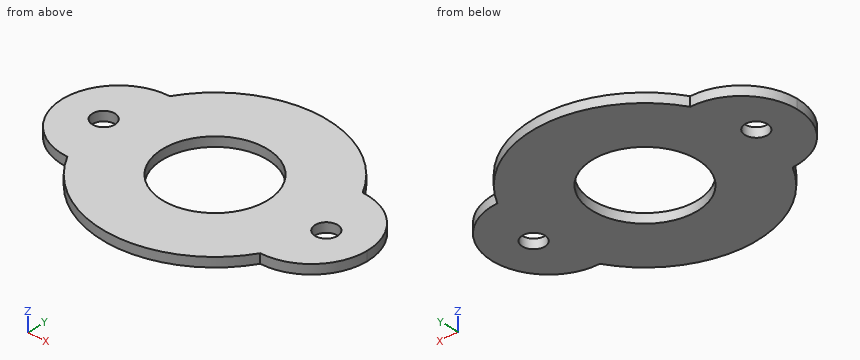
from build123d import *

# Parameters (mm, degrees)
F0_R     = 7
F1_DEPTH = 1.25
F2_R     = 7.49999
F3_D     = 3


# Not quite as in the source:
# - a fillet or chamfer is up to 0.001 mm smaller than in the source, because OpenCascade refuses the exact size


with BuildPart() as f1:
    # F0 (on Top) → F1 (new body)
    with BuildSketch(Plane.XY):
        with BuildLine():
            ThreePointArc((-12.990381, -7.5), (-15, 0), (-12.990381, 7.5))
            Line((-12.990381, 7.5), (-20.490381, 7.5))
            Line((-20.490381, 7.5), (-20.490381, -7.5))
            Line((-20.490381, -7.5), (-12.990381, -7.5))
        make_face()
        with BuildLine():
            ThreePointArc((12.990381, -7.5), (14.488887, -3.882286), (15, 0))
            ThreePointArc((15, 0), (14.488887, 3.882286), (12.990381, 7.5))
            ThreePointArc((12.990381, 7.5), (0, 15), (-12.990381, 7.5))
            ThreePointArc((-12.990381, 7.5), (-15, 0), (-12.990381, -7.5))
            ThreePointArc((-12.990381, -7.5), (0, -15), (12.990381, -7.5))
        make_face()
        Circle(F0_R, mode=Mode.SUBTRACT)
        with BuildLine():
            ThreePointArc((12.990381, 7.5), (14.488887, 3.882286), (15, 0))
            ThreePointArc((15, 0), (14.488887, -3.882286), (12.990381, -7.5))
            Line((12.990381, -7.5), (20.490381, -7.5))
            Line((20.490381, -7.5), (20.490381, 7.5))
            Line((20.490381, 7.5), (12.990381, 7.5))
        make_face()
    extrude(amount=F1_DEPTH)

    # F2 (radius 7.5 in the source; OpenCascade refuses exactly that, so slightly less here)
    f2_edges = [f1.edges().sort_by_distance(p)[0] for p in [
        (-20.490381, 7.5, 0.625),
        (-20.490381, -7.5, 0.625),
        (20.490381, 7.5, 0.625),
        (20.490381, -7.5, 0.625),
    ]]
    fillet(f2_edges, radius=F2_R)

    # F3 (through all)
    with Locations(Plane(origin=(0, 0, 0), x_dir=(1, 0, 0), z_dir=(0, 0, -1))):
        with Locations((15, 0), (-15, 0)):
            Hole(F3_D / 2)


solid = f1.part
CAD build for the part. Positions are in the model's coordinates, mm. Coordinates: 2 decimals unless noted, no trailing zeros. Write each loop counter-clockwise with the first axis right and the second up, starting at its lowest first coordinate (ties: lowest second). Pieces come first, ordered by that corner, then holes. Notation, with made-up numbers: M 6,53.25 L 14,53.25 A24 cw 14,78.25 Z; hole C 10,53.25 d6. An arc over 180 degrees is marked long. Answer as a JSON object with one key per item and string values. Group by question number.
1) Pin check, flat tip, straight feed: pin 1 Ø3 at (x, y) = (-7, 11.5) entering from -Z. Stop position of the tip, or through.
2) Saw through at A-A (x = 0). Write the cut outline in (y, z).
3) Saw through at C-C (y = 12). Write the cut outline in (x, z), plus the area to 3 significant figures.
4) Saw through at B-B (z = 0.5). Give the number of separate pieces and of enclosed holes in the cut face, plus the area to 3 significant figures.
5) Saw through at D-D (x = -4.5). Write the cut outline in (y, z), plus the area to 3 significant figures.
6) Wall check: line 1 (X direction, y = -0.5, z = 0.25); line 2 (Y direction, x = -13, z = 0.1); line 3 (Y direction, x = 15, z = 0.9). Give the ranges that are in metal, low to high. Write a range as from..to.
Values follow:
{
 "1": {"pin 1": "stops at z = 0"},
 "2": {"outline": "M -15,0 L -7,0 L -7,1.25 L -15,1.25 Z; M 7,0 L 15,0 L 15,1.25 L 7,1.25 Z"},
 "3": {"outline": "M -9,0 L 9,0 L 9,1.25 L -9,1.25 Z", "area": "22.5 mm2"},
 "4": {"separate pieces": "1", "enclosed holes": "3", "area": "675 mm2"},
 "5": {"outline": "M -14.31,0 L -5.36,0 L -5.36,1.25 L -14.31,1.25 Z; M 5.36,0 L 14.31,0 L 14.31,1.25 L 5.36,1.25 Z", "area": "22.4 mm2"},
 "6": {"line 1": "x = -20.47..-16.41, -13.59..-6.98, 6.98..13.59, 16.41..20.47", "line 2": "y = -7.5..7.5", "line 3": "y = -7.23..-1.5, 1.5..7.23"}
}
